Input: part model. Units: mm. Frame: model coordinates. Face numbers are marked on the shaded views. A direction names the side the tool comes from. Round coordinates to 2 decimals unless told otherwise and drop trailing zeros. Loops run counter-clockwise (first coordinate to the right, second up) from the corner with the lowest first, then second, coordinate; pieces in that order, holes last. Notation, with made-up numbers: (80, -30) -> (88, -30) arc R21 cw to (88, -15) -> close; hole circle Ø2 at (35, 75). An arc over 180 degrees is marked (long way). Answer as a JSON object with one key per item and string values.
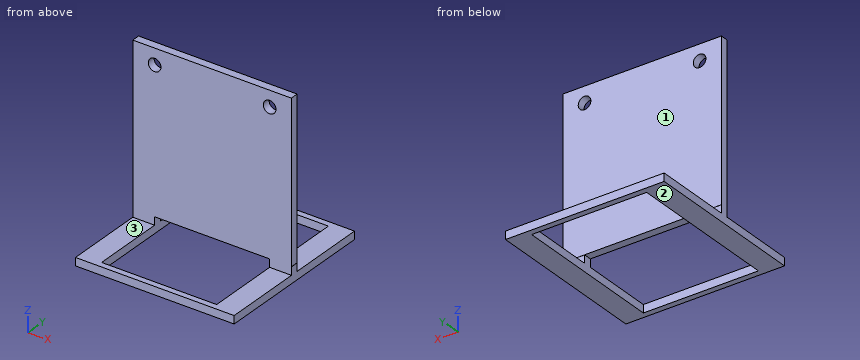
```python
from build123d import *

# Parameters (mm, degrees)
F0_W     = 40
F0_H     = 42
F0_W_2   = 29
F0_H_2   = 39
F1_DEPTH = 2
F2_W     = 5.5
F2_H     = 2
F3_DEPTH = 2
F4_W     = 5.5
F4_H     = 2
F5_DEPTH = 40
F6_R     = 1.594694
F7_DEPTH = 3


with BuildPart() as f1:
    # F0 (on Top) → F1 (new body)
    with BuildSketch(Plane.XY):
        Rectangle(F0_W, F0_H)
        Rectangle(F0_W_2, F0_H_2, mode=Mode.SUBTRACT)
    extrude(amount=F1_DEPTH)

    # F2 (on face) → F3 (join)
    with BuildSketch(Plane.XY.offset(2)):
        with Locations((-17.25, 0)):
            Rectangle(F2_W, F2_H)
        with Locations((17.25, 0)):
            Rectangle(F2_W, F2_H)
    extrude(amount=F3_DEPTH)

    # F4 (on face) → F5 (join)
    with BuildSketch(Plane.XY.offset(4)):
        Polygon((-14.5, 1), (-14.5, -1), (19.954836, -1), (19.954836, 1.025821), (-20, 1.025821), (-20, 1), align=None)
        with Locations((-17.25, 0)):
            Rectangle(F4_W, F4_H)
    extrude(amount=F5_DEPTH)

    # F6 (on face) → F7 (cut)
    with BuildSketch(Plane.XZ.offset(1)):
        with Locations((-14.5, 40)):
            Circle(F6_R)
        with Locations((14.5, 40)):
            Circle(F6_R)
    extrude(amount=-F7_DEPTH, mode=Mode.SUBTRACT)


solid = f1.part
```
1) Ray query, probe 1 along Y at (x, z) = (-10, 30.5); probe 2 along Z at (x, y) = (-16, 6); probe 3 along Z at (x, y) = (12.5, -0.5). Return the intervals inside material, ascending.
Output:
{"probe 1": "y = -1 to 1.03", "probe 2": "z = 0 to 2", "probe 3": "z = 4 to 44"}
2) Section C-C, the plane x = -10.5. Output: boundary loops of the cut face in (y, z).
Output:
{"outline": "(-21, 0) -> (-19.5, 0) -> (-19.5, 2) -> (-21, 2) -> close; (-1, 4) -> (1.03, 4) -> (1.03, 44) -> (-1, 44) -> close; (19.5, 0) -> (21, 0) -> (21, 2) -> (19.5, 2) -> close"}
3) Reachability of the marked faces 1, 2 and 3 from +Z, -Z, +X, -X, +Y, -Y: full face, straight path, thin tool, end or side. Return the list, or none.
Output:
{"face 1": "+Z, +X, -X, +Y", "face 2": "-Z, +X, -X, +Y, -Y", "face 3": "+Z, +X, -X, -Y"}
4) Section D-D, the plane z = 24.5. Output: boundary loops of the cut face in (x, y), plus the area to 3 significant figures.
Output:
{"outline": "(-20, -1) -> (19.95, -1) -> (19.95, 1.03) -> (-20, 1.03) -> close", "area": "80.9 mm^2"}
5) Section B-B, the plane z = 40. Output: boundary loops of the cut face in (x, y), plus the area to 3 significant figures.
Output:
{"outline": "(-20, -1) -> (-16.09, -1) -> (-16.09, 1.03) -> (-20, 1.03) -> close; (-12.91, -1) -> (12.91, -1) -> (12.91, 1.03) -> (-12.91, 1.03) -> close; (16.09, -1) -> (19.95, -1) -> (19.95, 1.03) -> (16.09, 1.03) -> close", "area": "68.0 mm^2"}
6) Section A-A, the plane y = -17.5. Output: boundary loops of the cut face in (x, z), plus the area to 3 significant figures.
Output:
{"outline": "(-20, 0) -> (-14.5, 0) -> (-14.5, 2) -> (-20, 2) -> close; (14.5, 0) -> (20, 0) -> (20, 2) -> (14.5, 2) -> close", "area": "22.0 mm^2"}
7) Contact query for flat-ended pins moving along their axis: P1, Ø4, axis at x = -14.5, z = 40, coming from the +Y side; P2, Ø10, axis at x = 4, y = 13.5, coming from the +Z side; P3, Ø4, axis at x = 14.5, z = 40, coming from the -Y side; P4, Ø12, axis at y = 1, z = 23.5, coming from the +X side. Output: stop coordinate, or through.
Output:
{"P1": "stops at y = 1.03", "P2": "passes through", "P3": "stops at y = -1", "P4": "stops at x = 19.95"}
